```python
from build123d import *

# Parameters (mm, degrees)
SKETCH1_R           = 10
BOSS_EXTRUDE1_DEPTH = 37
SKETCH2_R           = 12.5
BOSS_EXTRUDE2_DEPTH = 2
SKETCH3_R           = 5
BOSS_EXTRUDE3_DEPTH = 30


with BuildPart() as part:
    # Sketch1 → Boss-Extrude1 (new body)
    with BuildSketch(Plane(origin=(0, 0, 0), x_dir=(0, 0, -1), z_dir=(1, 0, 0))):
        Circle(SKETCH1_R)
    boss_extrude1 = extrude(amount=BOSS_EXTRUDE1_DEPTH)

    # Sketch2 → Boss-Extrude2 (add)
    with BuildSketch(Plane(origin=(37, 0, 0), x_dir=(0, 0, -1), z_dir=(1, 0, 0))):
        Circle(SKETCH2_R)
    boss_extrude2 = extrude(amount=BOSS_EXTRUDE2_DEPTH)

    # Sketch3 → Boss-Extrude3 (add)
    with BuildSketch(Plane(origin=(39, 0, 0), x_dir=(0, 0, -1), z_dir=(1, 0, 0))):
        Circle(SKETCH3_R)
    boss_extrude3 = extrude(amount=BOSS_EXTRUDE3_DEPTH)

    # Mirror2: Boss-Extrude1, Boss-Extrude2, Boss-Extrude3 across plane
    add(boss_extrude1.mirror(Plane(origin=(0, 0, 0), x_dir=(0, 0, 1), z_dir=(1, 0, 0))))
    add(boss_extrude2.mirror(Plane(origin=(0, 0, 0), x_dir=(0, 0, 1), z_dir=(1, 0, 0))))
    add(boss_extrude3.mirror(Plane(origin=(0, 0, 0), x_dir=(0, 0, 1), z_dir=(1, 0, 0))))


solid = part.part
```
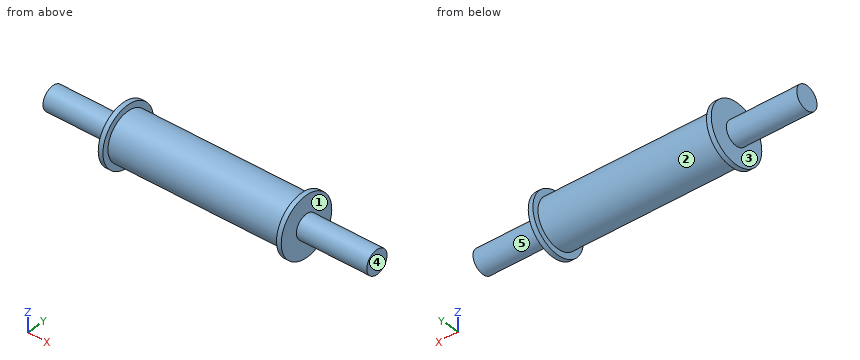
Here's how the part is built. I have some questions about the finished solid (model axes, mm). Face numbers are marked on the shaded views. A direction names the side the tool comes from. Round coordinates to 2 decimals unless told otherwise and drop trailing zeros. Write each loop counter-clockwise with the first axis right and the second up, starting at its lowest first coordinate (ties: lowest second). Pieces come first, ordered by that corner, then holes.
Q1. If we section it at D-D on x = 56: Write out the boundary of the cut face in (y, z).
Q2. If we section it at A-A on y = 0: Write out the boundary of the cut face in (x, z), plus the area to 3 significant figures.
Q3. Which directions (+Z, -Z, +X, -X, +Y, -Y) give clear straight access to the entire face, cutting with the end or side of a thin tool? Please do the marked faces 3, 4 and 5.
Q4. If we section it at C-C on x = -3: Write out the boundary of the cut face in (y, z).
Q5. If we mould it in two halves opening along Z, with no side actions, what happens to the marked faces 1 and 2? For each: +Z half, -Z half, draft (parallel to the pull), parting line (faces both ways), or undercut.
Q6. Please list where these lines run through material, in increasing order: probe 1 along X at (y, z) = (8.75, 6.25); probe 2 along X at (y, z) = (4.25, -8); probe 3 along Z at (x, y) = (60, 0.25).
Q7. Will these pins go through, and if not, where does the flat tip stop? P1, Ø8, axis at x = -32.5, z = -4, coming from the -Y side; P2, Ø5, axis at x = 53, y = -2.5, coming from the +Z side; P3, Ø12, axis at x = 8.5, z = 10, coming from the -Y side; P4, Ø7.5, axis at y = 2, z = -6, coming from the -X side.
Answer below:
1. outline: circle Ø10 at (0, 0)
2. outline: (-69, -5) - (-39, -5) - (-39, -12.5) - (-37, -12.5) - (-37, -10) - (37, -10) - (37, -12.5) - (39, -12.5) - (39, -5) - (69, -5) - (69, 5) - (39, 5) - (39, 12.5) - (37, 12.5) - (37, 10) - (-37, 10) - (-37, 12.5) - (-39, 12.5) - (-39, 5) - (-69, 5) - close
2. area: 2,180 mm2
3. face 3: -X
3. face 4: +Z, -Z, +X, +Y, -Y
3. face 5: +X
4. outline: circle Ø20 at (0, 0)
5. face 1: draft
5. face 2: parting line
6. probe 1: x = -39 to -37, 37 to 39
6. probe 2: x = -39 to 39
6. probe 3: z = -4.99 to 4.99
7. P1: stops at y = -10
7. P2: stops at z = 5
7. P3: stops at y = -9.17
7. P4: stops at x = -69
